Design review of the part built by this model. Coordinates are the model's own, in mm. A direction names the side the tool comes from. Coordinates: 2 decimals unless noted, no trailing zeros. Loops run counter-clockwise (first coordinate to the right, second up) from the corner with the lowest first, then second, coordinate; pieces in that order, holes last. Notation, with made-up numbers: (72.25, 56) -> (82.25, 56) arc R18 ccw to (82.25, 69) -> close; hole circle Ø4 at (-24.5, 32.5). An arc over 180 degrees is marked (long way). Use one line per item in the form item = value. Start each with the question number.
1. Consider section D-D (z = 17.25). State the section outline as (x, y) points, then the cut area to 3 significant figures.
2. Machinability: for faces 4 (the face through (0, 0, 5)), 5 (the face through (0, -2, 23)), 6 (the face through (3.045, -1.726, 12.675)), which of the approach directions +Z, -Z, +X, -X, +Y, -Y give a long, thin tool a straight path to every point of the face, cutting with its end or side? Answer none if there is none.
3. Consider section B-B (z = 3.75). State the section outline as (x, y) points.
4. The part is to be moulded in two halves that separate along Y. For faces 1 (the face through (0, 3.5, 13)), 2 (the face through (0, 0, 20)), 3 (the face through (0, -3.5, 13)), say which applies: released by +Y, released by -Y, zero draft, split by the parting line, or undercut.
5. Consider section C-C (y = -1.5). State the section outline as (x, z) points, then the cut area to 3 significant figures.
6. For pin 1 (3 mm diameter, centred on x = 0.5, y = 0.5, fed in from +Z); pin 2 (3.5 mm diameter, centred on x = 0, y = 0, fed in from +Z); pin 3 (2.5 mm diameter, centred on x = 0, y = 0, fed in from -Z); pin 4 (2 mm diameter, centred on y = -0.5, z = 15, fed in from +X), all flat-tipped, find the tip position at first contact; note any pin that passes through.
7. Wall thickness on line 1 (Y direction, x = 0, z = 3.5); line 2 (Z direction, x = 0.75, y = 1); line 3 (X direction, y = 1.5, z = 20.5): over which ranges is each line inside the solid? List them lowest first. Write a range as from..to.
8. Consider section A-A (x = 0). State the section outline as (y, z) points.
Autodesk Inventor part; units mm, degrees
ref_plane "YZ Plane" through (0, 0, 0) normal (1, 0, 0) x (0, 1, 0)
ref_plane "XZ Plane" through (0, 0, 0) normal (0, 1, 0) x (-1, 0, 0)
ref_plane "XY Plane" through (0, 0, 0) normal (0, 0, 1) x (1, 0, 0)
sketch "Sketch1" plane through (0, 0, 0) normal (0, 0, 1) x (1, 0, 0)
  circle A0 centre (0, 0) radius 4.5
  dimension "d0" = 9
extrude "Extrusion1" add sketch "Sketch1" along normal blind 25
sketch "Sketch2" plane through (0, 0, 25) normal (0, 0, 1) x (1, 0, 0)
  circle A0 centre (0, 0) radius 2
  dimension "d3" = 4
extrude "Extrusion2" cut sketch "Sketch2" against normal blind 5
sketch "Sketch3" plane through (0, 0, 0) normal (0, 0, -1) x (-1, 0, 0)
  circle A0 centre (0, 0) radius 2
  dimension "d6" = 4
extrude "Extrusion3" cut sketch "Sketch3" against normal blind 5
sketch "Sketch4" plane through (0, 0, 25) normal (0, 0, 1) x (1, 0, 0)
  line L0 (2.0207, 3.5) -> (4.0415, 0)
  line L1 (4.0415, 0) -> (2.0207, -3.5)
  line L2 (2.0207, -3.5) -> (-2.0207, -3.5)
  line L3 (-2.0207, -3.5) -> (-4.0415, 0)
  line L4 (-4.0415, 0) -> (-2.0207, 3.5)
  line L5 (-2.0207, 3.5) -> (2.0207, 3.5)
  circle A0 centre (0, 0) radius 4.5
  dimension "d9" = 7
extrude "Extrusion4" cut sketch "Sketch4" against normal up to surface (25 mm away)
properties part number "CapacitorBankStandoff"
Geometry check:
q1.outline = (-4.04, 0) -> (-2.02, -3.5) -> (2.02, -3.5) -> (4.04, 0) -> (2.02, 3.5) -> (-2.02, 3.5) -> close
q1.area = 42.4 mm²
q2.face_4 = -Z
q2.face_5 = +Z
q2.face_6 = +Z, -Z, +X, -Y
q3.outline = (-4.04, 0) -> (-2.02, -3.5) -> (2.02, -3.5) -> (4.04, 0) -> (2.02, 3.5) -> (-2.02, 3.5) -> close; hole circle Ø4 at (0, 0)
q4.face_1 = released by +Y
q4.face_2 = undercut
q4.face_3 = released by -Y
q5.outline = (-3.18, 0) -> (-1.32, 0) -> (-1.32, 5) -> (1.32, 5) -> (1.32, 0) -> (3.18, 0) -> (3.18, 25) -> (1.32, 25) -> (1.32, 20) -> (-1.32, 20) -> (-1.32, 25) -> (-3.18, 25) -> close
q5.area = 132 mm²
q6.pin_1 = 25
q6.pin_2 = 20
q6.pin_3 = 5
q6.pin_4 = 4.04
q7.line_1 = -3.5..-2, 2..3.5
q7.line_2 = 5..20
q7.line_3 = -3.18..-1.32, 1.32..3.18
q8.outline = (-3.5, 0) -> (-2, 0) -> (-2, 5) -> (2, 5) -> (2, 0) -> (3.5, 0) -> (3.5, 25) -> (2, 25) -> (2, 20) -> (-2, 20) -> (-2, 25) -> (-3.5, 25) -> close
